from build123d import *

# Parameters (mm, degrees)
SKETCH_1_R               = 2.1
SKETCH_1_W               = 40.5
SKETCH_1_H               = 20.5
SKETCH_1_R_2             = 6
EXTRUDE_1_DEPTH          = 3
SKETCH_2_R               = 3
SKETCH_2_R_2             = 2.1
CUT_EXTRUDE_1_DEPTH      = 10
SKETCH_3_R               = 1.5
CUT_EXTRUDE_2_DEPTH      = 10
SKETCH_4_R               = 2.1
CUT_EXTRUDE_3_DEPTH      = 10
CHAMFER_1_SIZE           = 10
FILLET_1_R               = 3
FILLET_2_R               = 2
SKETCH_5_R               = 2.1
CUT_EXTRUDE_4_DEPTH      = 10
CUT_EXTRUDE_5_DEPTH      = 10
MOVE_START               = 3
MOVE_FACE_1_OUTLINE_R    = 2.1
MOVE_FACE_1_DEPTH        = 144
FILLET_3_R               = 2
DELETE_START             = -3
DELETE_FACE_1_DEPTH      = 150
DELETE_FACE_2_OUTLINE_R  = 2.1
DELETE_FACE_2_DEPTH      = 150
CUT_EXTRUDE_6_DEPTH      = 177.068168617
CUT_EXTRUDE_6_DEPTH_BACK = 177.068168617
FILLET_4_R               = 5
FILLET_5_R               = 1


# Read off the part's stored shape, not the designer's step: 移动面1, 删除面1, 删除面2
with BuildPart() as part:
    # 草图1 → 凸台-拉伸1 (new, symmetric)
    with BuildSketch(Plane(origin=(0, 0, 0), x_dir=(0, 0, -1), z_dir=(1, 0, 0))):
        with BuildLine():
            Line((-60, -42.021540511), (0, -70))
            Line((0, -70), (12, -70))
            Line((12, -70), (12, 30))
            Line((12, 30), (-75.715728753, 30))
            Line((-75.715728753, 30), (-125.857864376, 80.142135624))
            ThreePointArc((-125.857864376, 80.142135624), (-154.142135624, 80.142135624), (-154.142135624, 51.857864376))
            Line((-154.142135624, 51.857864376), (-92.284271247, -10))
            Line((-92.284271247, -10), (-60, -10))
            Line((-60, -10), (-60, -42.021540511))
        make_face()
        with Locations((-73.77114317, 0.625)):
            Circle(SKETCH_1_R, mode=Mode.SUBTRACT)
        with Locations((-49.02114317, 5.625)):
            Rectangle(SKETCH_1_W, SKETCH_1_H, mode=Mode.SUBTRACT)
        with Locations((-24.27114317, 0.625)):
            Circle(SKETCH_1_R, mode=Mode.SUBTRACT)
        Circle(SKETCH_1_R_2, mode=Mode.SUBTRACT)
        with Locations((-73.77114317, 10.625)):
            Circle(SKETCH_1_R, mode=Mode.SUBTRACT)
        with Locations((-24.27114317, 10.625)):
            Circle(SKETCH_1_R, mode=Mode.SUBTRACT)
    extrude(amount=EXTRUDE_1_DEPTH, both=True)

    # 草图2 → 切除-拉伸1 (cut)
    with BuildSketch(Plane(origin=(3, 0, 0), x_dir=(0, 0, -1), z_dir=(1, 0, 0))):
        with Locations((-140, 66)):
            Circle(SKETCH_2_R)
        with Locations((-140, 82)):
            Circle(SKETCH_2_R_2)
        with Locations((-126.143593539, 74)):
            Circle(SKETCH_2_R_2)
        with Locations((-126.143593539, 58)):
            Circle(SKETCH_2_R_2)
        with Locations((-140, 50)):
            Circle(SKETCH_2_R_2)
        with Locations((-153.856406461, 58)):
            Circle(SKETCH_2_R_2)
        with Locations((-153.856406461, 74)):
            Circle(SKETCH_2_R_2)
    extrude(amount=-CUT_EXTRUDE_1_DEPTH, mode=Mode.SUBTRACT)

    # 草图3 → 切除-拉伸2 (cut)
    with BuildSketch(Plane(origin=(3, 0, 0), x_dir=(0, 0, -1), z_dir=(1, 0, 0))):
        with Locations((-69.27114317, 15.875)):
            Circle(SKETCH_3_R)
        with Locations((-28.77114317, 15.875)):
            Circle(SKETCH_3_R)
        with Locations((-69.27114317, -4.625)):
            Circle(SKETCH_3_R)
        with Locations((-28.77114317, -4.625)):
            Circle(SKETCH_3_R)
    extrude(amount=-CUT_EXTRUDE_2_DEPTH, mode=Mode.SUBTRACT)

    # 草图4 → 切除-拉伸3 (cut)
    with BuildSketch(Plane(origin=(3, 0, 0), x_dir=(0, 0, -1), z_dir=(1, 0, 0))):
        with Locations((-55, -15)):
            Circle(SKETCH_4_R)
        with Locations((-55, -35)):
            Circle(SKETCH_4_R)
        with Locations((7, -65)):
            Circle(SKETCH_4_R)
        with Locations((7, -45)):
            Circle(SKETCH_4_R)
        with Locations((-8, -60.75264914)):
            Circle(SKETCH_4_R)
        with Locations((-26.126155741, -52.300283905)):
            Circle(SKETCH_4_R)
        with Locations((-44.252311481, -43.84791867)):
            Circle(SKETCH_4_R)
    extrude(amount=-CUT_EXTRUDE_3_DEPTH, mode=Mode.SUBTRACT)

    # 倒角1
    chamfer_1_edges = [part.edges().sort_by_distance(p)[0] for p in [
        (0, -10, 60),
    ]]
    chamfer(chamfer_1_edges, length=CHAMFER_1_SIZE)

    # 圆角1
    fillet_1_edges = [part.edges().sort_by_distance(p)[0] for p in [
        (0, -20, 60),
        (0, -10, 70),
        (0, 30, -12),
        (0, -70, -12),
        (0, -70, 0),
        (0, -42.021540511, 60),
        (0, -10, 92.284271247),
        (0, 30, 75.715728753),
    ]]
    fillet(fillet_1_edges, radius=FILLET_1_R)

    # 圆角2
    fillet_2_edges = [part.edges().sort_by_distance(p)[0] for p in [
        (0, 15.875, 30.27114317),
        (0, 14.375, 28.77114317),
        (0, -4.625, 67.77114317),
        (0, -3.125, 69.27114317),
        (0, -4.625, 30.27114317),
        (0, -3.125, 28.77114317),
        (0, 14.375, 69.27114317),
        (0, 15.875, 67.77114317),
    ]]
    fillet(fillet_2_edges, radius=FILLET_2_R)

    # 草图5 → 切除-拉伸4 (cut)
    with BuildSketch(Plane(origin=(3, 0, 0), x_dir=(0, 0, -1), z_dir=(1, 0, 0))):
        with Locations((-110, 57.213203436)):
            Circle(SKETCH_5_R)
        with Locations((-88.786796564, 36)):
            Circle(SKETCH_5_R)
        with Locations((-109.946763354, 14.785654888)):
            Circle(SKETCH_5_R)
        with Locations((-131.214342006, 35.94434337)):
            Circle(SKETCH_5_R)
        with Locations((-62.230447378, 25)):
            Circle(SKETCH_5_R)
        with Locations((-32.230447378, 25)):
            Circle(SKETCH_5_R)
    extrude(amount=-CUT_EXTRUDE_4_DEPTH, mode=Mode.SUBTRACT)

    # 草图6 → 切除-拉伸5 (cut)
    with BuildSketch(Plane(origin=(3, 0, 0), x_dir=(0, 0, -1), z_dir=(1, 0, 0))):
        with BuildLine():
            ThreePointArc((-60.878679656, -19.121320344), (-60.228361402, -20.09459039), (-60, -21.242640687))
            Line((-60, -21.242640687), (-60, -10))
            Line((-60, -10), (-50, -10))
            Line((-50, -10), (-50, -21.242640687))
            Line((-50, -21.242640687), (-50, -35.650837903))
            Line((-50, -35.650837903), (2.216946626, -60))
            Line((2.216946626, -60), (9, -60))
            Line((9, -60), (12, -60))
            Line((12, -60), (12, 27))
            ThreePointArc((12, 27), (11.121320344, 29.121320344), (9, 30))
            Line((9, 30), (-74.473088065, 30))
            ThreePointArc((-74.473088065, 30), (-75.621138363, 30.228361402), (-76.594408409, 30.878679656))
            Line((-76.594408409, 30.878679656), (-125.857864376, 80.142135624))
            ThreePointArc((-125.857864376, 80.142135624), (-154.142135624, 80.142135624), (-154.142135624, 51.857864376))
            Line((-154.142135624, 51.857864376), (-93.162950904, -9.121320344))
            ThreePointArc((-93.162950904, -9.121320344), (-92.189680857, -9.771638598), (-91.04163056, -10))
            Line((-91.04163056, -10), (-71.242640687, -10))
            ThreePointArc((-71.242640687, -10), (-70.09459039, -10.228361402), (-69.121320344, -10.878679656))
            Line((-69.121320344, -10.878679656), (-60.878679656, -19.121320344))
        make_face()
    extrude(amount=-CUT_EXTRUDE_5_DEPTH, mode=Mode.SUBTRACT)

    # Move Face 1 outline → Move Face 1 (add)
    with BuildSketch(Plane.YZ.offset(MOVE_START)):
        with BuildLine():
            Line((-10, 60), (-40.110329728, 60))
            ThreePointArc((-40.110329728, 60), (-41.722228553, 59.530174337), (-42.829253089, 58.267854785))
            Line((-42.829253089, 58.267854785), (-69.718923361, 0.602770797))
            ThreePointArc((-69.718923361, 0.602770797), (-69.928888021, -0.015765146), (-70, -0.665083988))
            Line((-70, -0.665083988), (-70, -9))
            ThreePointArc((-70, -9), (-69.121320344, -11.121320344), (-67, -12))
            Line((-67, -12), (-60, -12))
            Line((-60, -12), (-60, -2.216946626))
            Line((-60, -2.216946626), (-35.650837903, 50))
            Line((-35.650837903, 50), (-10, 50))
            Line((-10, 50), (-10, 60))
        make_face()
        with Locations((-65, -7)):
            Circle(MOVE_FACE_1_OUTLINE_R, mode=Mode.SUBTRACT)
        with Locations((-60.75264914, 8)):
            Circle(MOVE_FACE_1_OUTLINE_R, mode=Mode.SUBTRACT)
        with Locations((-52.300283905, 26.126155741)):
            Circle(MOVE_FACE_1_OUTLINE_R, mode=Mode.SUBTRACT)
        with Locations((-43.84791867, 44.252311481)):
            Circle(MOVE_FACE_1_OUTLINE_R, mode=Mode.SUBTRACT)
        with Locations((-35, 55)):
            Circle(MOVE_FACE_1_OUTLINE_R, mode=Mode.SUBTRACT)
        with Locations((-15, 55)):
            Circle(MOVE_FACE_1_OUTLINE_R, mode=Mode.SUBTRACT)
    extrude(amount=MOVE_FACE_1_DEPTH)

    # 圆角3
    fillet_3_edges = [part.edges().sort_by_distance(p)[0] for p in [
        (72, -60, -12),
        (75, -60, -2.216946626),
        (75, -35.650837903, 50),
        (72, -10, 50),
        (72, -10, 60),
    ]]
    fillet(fillet_3_edges, radius=FILLET_3_R)

    # Delete Face 1 outline → Delete Face 1 (add)
    with BuildSketch(Plane.YZ.offset(DELETE_START)):
        with BuildLine():
            ThreePointArc((-60, -10), (-60.585786438, -11.414213562), (-62, -12))
            Line((-62, -12), (-60, -12))
            Line((-60, -12), (-60, -10))
        make_face()
        with BuildLine():
            Line((-70, -9), (-70, -12))
            Line((-70, -12), (-67, -12))
            ThreePointArc((-67, -12), (-69.121320344, -11.121320344), (-70, -9))
        make_face()
    extrude(amount=DELETE_FACE_1_DEPTH)

    # Delete Face 2 outline → Delete Face 2 (add)
    with BuildSketch(Plane.YZ.offset(DELETE_START)):
        with Locations((-65, -7)):
            Circle(DELETE_FACE_2_OUTLINE_R)
    extrude(amount=DELETE_FACE_2_DEPTH)

    # 草图8 → 切除-拉伸6 (cut, two sides: drawn at the far end of the back side and taken through both)
    with BuildSketch(Plane(origin=(147, 0, 0), x_dir=(0, 0, -1), z_dir=(1, 0, 0)).offset(-CUT_EXTRUDE_6_DEPTH_BACK)):
        with BuildLine():
            Line((-23.515068548, -48.000964265), (12, -67.8))
            Line((12, -67.8), (12, -60))
            Line((12, -60), (2.660335952, -60))
            ThreePointArc((2.660335952, -60), (2.227456724, -59.952592014), (1.815099428, -59.812615574))
            Line((1.815099428, -59.812615574), (-23.515068548, -48.000964265))
        make_face()
    extrude(amount=CUT_EXTRUDE_6_DEPTH + CUT_EXTRUDE_6_DEPTH_BACK, mode=Mode.SUBTRACT)

    # 圆角4
    # the kernel refuses this fillet: 5 mm, written as the material it takes off along each edge
    with BuildSketch(Plane(origin=(-10.171790934, -67.8, -12), x_dir=(0, 0.4869286506241587, 0.8734417491746865), z_dir=(1, 0, 0))) as fillet_4_piece_1:
        with BuildLine():
            CenterArc((2.868716374, 5), FILLET_4_R, 218.001756319, 51.998243681)
            Line((-1.071243031, 1.921571848), (-1.150042219, 1.860003285))
            ThreePointArc((-1.150042219, 1.860003285), (-0.622965691, 0.912093059), (-0.087344175, -0.048692865))
            Line((-0.087344175, -0.048692865), (0, -0.1))
            Line((0, -0.1), (2.868716374, -0.1))
            Line((2.868716374, -0.1), (2.868716374, 0))
        make_face()
    extrude(amount=164.343581869, mode=Mode.SUBTRACT)

    # 圆角5
    fillet_5_edges = [part.edges().sort_by_distance(p)[0] for p in [
        (72, -70, -12),
    ]]
    fillet(fillet_5_edges, radius=FILLET_5_R)


solid = part.part
Geometry check sheet. Reference: the model listing, model coordinates, mm. A direction names the side the tool comes from. Coordinates: 2 decimals unless noted, no trailing zeros. Loops run counter-clockwise (first coordinate to the right, second up) from the corner with the lowest first, then second, coordinate; pieces in that order, holes last. Notation, with made-up numbers: (78, -31.75) - (124, -31.75) arc R19 cw to (124, -16.75) - close; hole circle Ø10 at (-15, 76.5). An arc over 180 degrees is marked (long way). Use one line per item in the form item = value. Start each with the question number.
Item 1: Gauge pin test, flat ends, axial feed: pin 1 (12 mm diameter, centred on x = 13.5, y = -35.5, fed in from -Z); pin 2 (1 mm diameter, centred on x = 84, y = -36, fed in from -Z); pin 3 (10 mm diameter, centred on x = 52.5, z = -1, fed in from +Y). Record the tip position at first contact, or that the pin passes through.
Item 2: Section check A-A, the plane y = -15. Enter the section's corners in (x, z), and give its area (3 significant figures).
Item 3: Thickness scan on probe 1 along Y at (x, z) = (27, 55); probe 2 along Z at (x, y) = (138, -21.5); probe 3 along Y at (x, z) = (33, 8). Record the ranges inside material, lowest first.
Item 4: Section check D-D, the plane y = -23.5. Enter the section's corners in (x, z), and give its area (3 significant figures).
Item 5: Section check B-B, the plane z = 8. Enter the section's corners in (x, y).
Item 6: Tool access check on faces 1 (the face through (71, -23, 50)), 2 (the face through (71, -70, -6)). Record the directions out of +Z, -Z, +X, -X, +Y, -Y that give a thin tool (end or side, any length) a straight path to the whole face; none if there is none.
Item 7: Mould release check, pull along Z, two halves, no side actions. Record for faces 3 (the face through (70.95, -57.073, 7.241)), 4 (the face through (71, -10, 55)), 5 (the face through (73.05, -42.064, 45.36)): +Z half, -Z half, draft (parallel to the pull), parting line (faces both ways), or undercut.
Item 8: Section check C-C, the plane x = 93. Enter the section's corners in (y, z), and give its area (3 significant figures).
Computed:
q1.pin_1 = 37.46
q1.pin_2 = 48.18
q1.pin_3 = -58.88
q2.outline = (-3, 50) - (147, 50) - (147, 52.9) - (-3, 52.9) - close; (-3, 57.1) - (147, 57.1) - (147, 60) - (-3, 60) - close
q2.area = 870 mm2
q3.probe_1 = -44.35 to -37.1, -32.9 to -17.1, -12.9 to -10
q3.probe_2 = 50 to 60
q3.probe_3 = -66.27 to -62.85, -58.65 to -56.65
q4.outline = (-3, 50) - (147, 50) - (147, 60) - (-3, 60) - close
q4.area = 1,500 mm2
q5.outline = (-3, -66.27) - (147, -66.27) - (147, -62.85) - (-3, -62.85) - close; (-3, -58.65) - (147, -58.65) - (147, -56.65) - (-3, -56.65) - close
q6.face_1 = -Z, +X, -X, +Y
q6.face_2 = +Z, -Z, +X, -X, -Y
q7.face_3 = -Z half
q7.face_4 = draft
q7.face_5 = undercut
q8.outline = (-70, -10.65) arc R1 ccw to (-68.56, -11.54) arc R5 ccw to (-66.4, -9.49) - (-48, 23.52) - (-36.19, 48.85) arc R2 cw to (-34.38, 50) - (-12, 50) arc R2 ccw to (-10, 52) - (-10, 58) arc R2 ccw to (-12, 60) - (-40.11, 60) arc R3 ccw to (-42.83, 58.27) - (-69.72, 0.6) arc R3 ccw to (-70, -0.67) - close; hole circle Ø4.2 at (-60.75, 8); hole circle Ø4.2 at (-52.3, 26.13); hole circle Ø4.2 at (-43.85, 44.25); hole circle Ø4.2 at (-35, 55); hole circle Ø4.2 at (-15, 55)
q8.area = 863 mm2
